Here's the drawing with two shaded views (mm, measured from the low corner). I have some questions. A direction names the side the tool comes from. Round coordinates to 2 decimals unless told otherwise and drop trailing zeros. Write each loop counter-clockwise with the first axis right and the second up, starting at its lowest first coordinate (ties: lowest second). Pieces come first, ordered by that corner, then holes. Notation, with made-up numbers: M 66,19 L 94,19 A18 cw 94,33 Z; hole C -33.75,-26 d1. An arc over 180 degrees is marked long. Use one line per item in the form item = value. Start each with the question number.
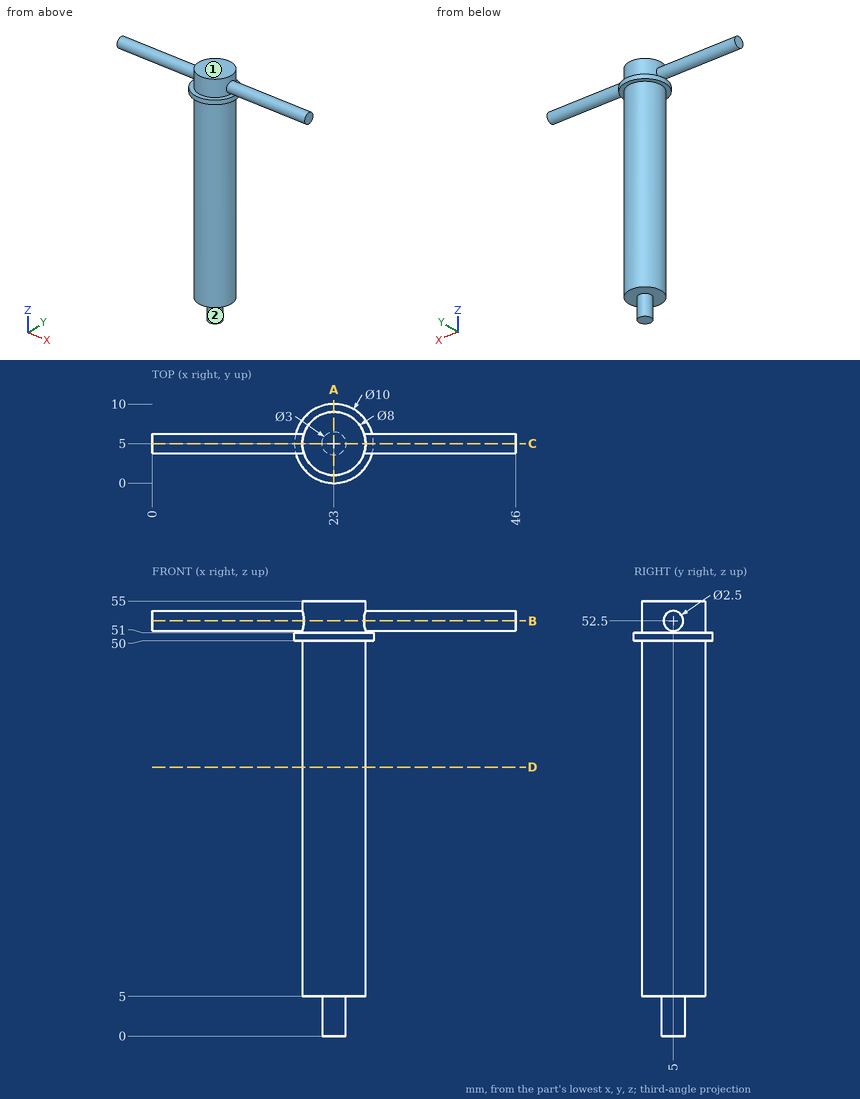
1. If we section it at D-D (z = 34): List the corners of the cut face in (x, y) for me.
2. If we section it at B-B (z = 52.5): List the corners of the cut face in (x, y) for me.
3. Please list where these lines run through material, in increasing order: line 1 along Z through (x, y) = (6, 5); line 2 along X through (y, z) = (5, 44.5); line 3 along Z through (x, y) = (23, 9.75).
4. If we section it at C-C (y = 5): List the corners of the cut face in (x, z) for me, and give its area (3 significant figures).
5. Will these pins go through, and if not, where does the flat tip stop? pin 1 (2 mm diameter, centred on y = 5, z = 36.5, fed in from -X); pin 2 (1.5 mm diameter, centred on x = 7, y = 3.5, fed in from +Z); pin 3 (3 mm diameter, centred on x = 18.5, y = 3, fed in from -Z).
6. Which directions (+Z, -Z, +X, -X, +Y, -Y) give clear straight access to the entire face, cutting with the end or side of a thin tool? Please do the marked faces 1 and 2.
7. If we section it at A-A (x = 23): List the corners of the cut face in (y, z) for me.
Model answer:
q1.outline = C 23,5 d8
q2.outline = M 0,3.75 L 19.2,3.75 A4 ccw 26.8,3.75 L 46,3.75 L 46,6.25 L 26.8,6.25 A4 ccw 19.2,6.25 L 0,6.25 Z
q3.line_1 = 51.25 to 53.75
q3.line_2 = 19 to 27
q3.line_3 = 50 to 51
q4.outline = M 0,51.25 L 19,51.25 L 19,51 L 18,51 L 18,50 L 19,50 L 19,5 L 21.5,5 L 21.5,0 L 24.5,0 L 24.5,5 L 27,5 L 27,50 L 28,50 L 28,51 L 27,51 L 27,51.25 L 46,51.25 L 46,53.75 L 27,53.75 L 27,55 L 19,55 L 19,53.75 L 0,53.75 Z
q4.area = 512 mm2
q5.pin_1 = 19
q5.pin_2 = 53.5
q5.pin_3 = 5
q6.face_1 = +Z, +X, -X, +Y, -Y
q6.face_2 = -Z
q7.outline = M 0,50 L 1,50 L 1,5 L 3.5,5 L 3.5,0 L 6.5,0 L 6.5,5 L 9,5 L 9,50 L 10,50 L 10,51 L 9,51 L 9,55 L 1,55 L 1,51 L 0,51 Z
